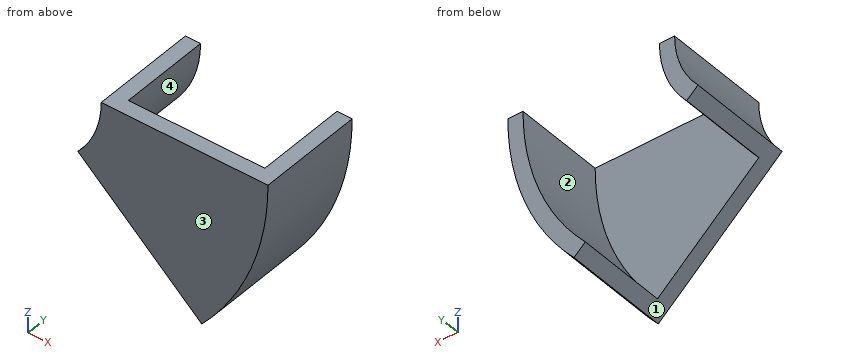
Autodesk Inventor part; units mm, degrees
ref_plane "YZ Plane" through (0, 0, 0) normal (1, 0, 0) x (0, 1, 0)
ref_plane "XZ Plane" through (0, 0, 0) normal (0, 1, 0) x (-1, 0, 0)
ref_plane "XY Plane" through (0, 0, 0) normal (0, 0, 1) x (1, 0, 0)
sketch "Sketch1" plane through (0, 0, 0) normal (0, 0, 1) x (1, 0, 0)
  line L0 (0, 0) -> (0, 50) construction
  line L1 (0, 50) -> (30, 50) construction
  line L2 (30, 50) -> (30, 15)
  line L3 (30, 15) -> (85, 15)
  line L4 (85, 15) -> (85, 50)
  line L5 (85, 50) -> (80, 50)
  line L6 (80, 50) -> (80, 20)
  line L7 (80, 20) -> (35, 20)
  line L8 (35, 20) -> (35, 50)
  line L9 (35, 50) -> (30, 50)
  dimension "d0" = 50
  dimension "d1" = 30
  dimension "d2" = 35
  dimension "d3" = 55
  dimension "d4" = 35
  dimension "d5" = 5
  dimension "d6" = 30
  dimension "d7" = 45
revolve "Revolution1" add sketch "Sketch1" angle 42 about axis through (0, 0, 0) along (0, 1, 0)
properties part number "track z2059"
Can you work these out from the model? Positions are in its coordinate system, mm. Face numbers are marked on the shaded views. Coordinates: 2 decimals unless noted, no trailing zeros. Write each loop counter-clockwise with the first axis right and the second up, starting at its lowest first coordinate (ties: lowest second). Pieces come first, ordered by that corner, then holes. Notation, with made-up numbers: (57.25, 27) - (77.25, 27) arc R16 ccw to (77.25, 40) - close; hole circle Ø6 at (75.25, 75). An arc over 180 degrees is marked (long way). Return JSON: item names as keys, results as strings.
Q1. If we section it at D-D (x = 74): Please give me the cut outline in (y, z), then the cut area to 3 significant figures.
Computed values:
{"outline": "(15, -41.82) - (50, -41.82) - (50, -30.4) - (20, -30.4) - (20, 0) - (15, 0) - close", "area": "552 mm2"}
Q2. I'm going to push flat-ended pins straight in: pin 1 Ø16 at (x, z) = (42.5, -38.5) entering from +Y; pin 2 Ø6 at (x, y) = (66, 33.5) entering from +Z; pin 3 Ø2 at (y, z) = (29, -11.5) entering from -X. Where does each tip first touch, or does it pass through?
Computed values:
{"pin 1": "stops at y = 20", "pin 2": "stops at z = -40.48", "pin 3": "stops at x = 27.27"}
Q3. If we section it at C-C (y = 18): Please give me the cut outline in (x, z).
Computed values:
{"outline": "(22.29, -20.07) - (63.17, -56.88) arc R85 ccw to (85, 0) - (30, 0) arc R30 cw to start"}
Q4. Thinking about a two-plate mould opening in X: for the marked faces 1, 2, 3 and 4, which applies, +X half, -X half, draft (parallel to the pull), parting line (faces both ways), or undercut?
Computed values:
{"face 1": "-X half", "face 2": "undercut", "face 3": "draft", "face 4": "undercut"}
Q5. If we section it at A-A (y = 43.5): Please give me the cut outline in (x, z), then the cut area to 3 significant figures.
Computed values:
{"outline": "(22.29, -20.07) - (26.01, -23.42) arc R35 ccw to (35, 0) - (30, 0) arc R30 cw to start; (59.45, -53.53) - (63.17, -56.88) arc R85 ccw to (85, 0) - (80, 0) arc R80 cw to start", "area": "421 mm2"}
Q6. Please list where these lines run through material, in increasing order: L1, parallel to Y at x = 61, z = -34.5; L2, parallel to X at y = 47.5, z = -5.5; L3, parallel to X at y = 42.5, z = -17. Write a range as from..to.
Computed values:
{"L1": "y = 15..20", "L2": "x = 29.49..34.57, 79.81..84.82", "L3": "x = 24.72..30.59, 78.17..83.28"}
Q7. If we section it at B-B (z = -6.5): Please give me the cut outline in (x, y), then the cut area to 3 significant figures.
Computed values:
{"outline": "(29.29, 15) - (84.75, 15) - (84.75, 50) - (79.74, 50) - (79.74, 20) - (34.39, 20) - (34.39, 50) - (29.29, 50) - close", "area": "581 mm2"}
